Source: CAD feature listing. Evaluate the final solid. Frame: model axes, mm. Coordinates: 2 decimals unless noted, no trailing zeros. Loops run counter-clockwise (first coordinate to the right, second up) from the corner with the lowest first, then second, coordinate; pieces in that order, holes last.
Item 1: Section query B-B, the plane y = 0.7. State how many separate pieces and enclosed holes the cut face has, then the cut area to 3 significant figures.
Item 2: Line query: probe 1 along Z at (x, y) = (1, 0.4). Output: solid intervals per line, ascending.
Item 3: Section query A-A, the plane x = 15. Return the cut outline in (y, z), then the cut area to 3 significant figures.
```python
from build123d import *

# Parameters (mm, degrees)
SKETCH1_W           = 22
SKETCH1_H           = 4
BOSS_EXTRUDE1_DEPTH = 1.5
SKETCH2_W           = 0.5
SKETCH2_H           = 0.5
CUT_EXTRUDE1_DEPTH  = 2
SKETCH3_R           = 0.01
CUT_EXTRUDE2_DEPTH  = 1.5


with BuildPart() as part:
    # Sketch1 → Boss-Extrude1 (new body)
    with BuildSketch(Plane(origin=(0, 0, 0), x_dir=(1, 0, 0), z_dir=(0, 1, 0))):
        with Locations((11, 2)):
            Rectangle(SKETCH1_W, SKETCH1_H)
    extrude(amount=BOSS_EXTRUDE1_DEPTH)

    # Sketch2 → Cut-Extrude1 (cut)
    with BuildSketch(Plane(origin=(0, 1.5, 0), x_dir=(1, 0, 0), z_dir=(0, 1, 0))):
        with Locations((3, 3)):
            Rectangle(SKETCH2_W, SKETCH2_H)
        with Locations((1, 3)):
            Rectangle(SKETCH2_W, SKETCH2_H)
        with Locations((5, 3)):
            Rectangle(SKETCH2_W, SKETCH2_H)
        with Locations((7, 3)):
            Rectangle(SKETCH2_W, SKETCH2_H)
        with Locations((9, 3)):
            Rectangle(SKETCH2_W, SKETCH2_H)
        with Locations((11, 3)):
            Rectangle(SKETCH2_W, SKETCH2_H)
        with Locations((13, 3)):
            Rectangle(SKETCH2_W, SKETCH2_H)
        with Locations((15, 3)):
            Rectangle(SKETCH2_W, SKETCH2_H)
        with Locations((17, 3)):
            Rectangle(SKETCH2_W, SKETCH2_H)
        with Locations((19, 3)):
            Rectangle(SKETCH2_W, SKETCH2_H)
        with Locations((21, 3)):
            Rectangle(SKETCH2_W, SKETCH2_H)
        with Locations((1, 1)):
            Rectangle(SKETCH2_W, SKETCH2_H)
        with Locations((3, 1)):
            Rectangle(SKETCH2_W, SKETCH2_H)
        with Locations((5, 1)):
            Rectangle(SKETCH2_W, SKETCH2_H)
        with Locations((7, 1)):
            Rectangle(SKETCH2_W, SKETCH2_H)
        with Locations((9, 1)):
            Rectangle(SKETCH2_W, SKETCH2_H)
        with Locations((11, 1)):
            Rectangle(SKETCH2_W, SKETCH2_H)
        with Locations((13, 1)):
            Rectangle(SKETCH2_W, SKETCH2_H)
        with Locations((15, 1)):
            Rectangle(SKETCH2_W, SKETCH2_H)
        with Locations((17, 1)):
            Rectangle(SKETCH2_W, SKETCH2_H)
        with Locations((19, 1)):
            Rectangle(SKETCH2_W, SKETCH2_H)
        with Locations((21, 1)):
            Rectangle(SKETCH2_W, SKETCH2_H)
    extrude(amount=-CUT_EXTRUDE1_DEPTH, mode=Mode.SUBTRACT)

    # Sketch3 → Cut-Extrude2 (cut)
    with BuildSketch(Plane(origin=(0, 1.5, 0), x_dir=(1, 0, 0), z_dir=(0, 1, 0))):
        with Locations(Location((11, 2, 0), (0, 0, 270))):
            Circle(SKETCH3_R)
    extrude(amount=-CUT_EXTRUDE2_DEPTH, mode=Mode.SUBTRACT)


solid = part.part
```
Verdict:
1. separate pieces: 1
1. enclosed holes: 23
1. area: 82.5 mm2
2. probe 1: z = -4 to -3.25, -2.75 to -1.25, -0.75 to 0
3. outline: (0, -4) - (1.5, -4) - (1.5, -3.25) - (0, -3.25) - close; (0, -2.75) - (1.5, -2.75) - (1.5, -1.25) - (0, -1.25) - close; (0, -0.75) - (1.5, -0.75) - (1.5, 0) - (0, 0) - close
3. area: 4.50 mm2
